Source: CAD feature listing. Evaluate the final solid. Frame: model axes, mm. Face numbers are marked on the shaded views. A direction names the side the tool comes from. Give positions to 0.01 mm unless a question says otherwise; leave off trailing zeros. Loops run counter-clockwise (first coordinate to the right, second up) from the corner with the lowest first, then second, coordinate; pieces in that order, holes last. Notation, with made-up numbers: (23.25, 0.25) -> (52.25, 0.25) arc R22 cw to (52.25, 8.25) -> close; hole circle Ø5 at (2.25, 69.5). An arc over 180 degrees is marked (long way). Return JSON: item names as keys, results as strings. Group by question number.
(1) Cut plane A-A on y = -11.9. Return loops of the section in (x, z) (3 decimals).
(2) Access query for the marked faces 1, 2 and 3. Directions: +Z, -Z, +X, -X, +Y, -Y. A direction counts if a zero-diameter tool reaches every point of the face in a straight line with its end or side. Return the directions, or none.
(3) Cut plane C-C on x = 2. Return loops of the section in (y, z).
(4) Cut plane B-B on z = 7. Return loops of the section in (x, y), then the cut area to 3 significant figures.
(5) Pin query (flat end, axial travel): pin 1 (3 mm diameter, centred on x = 3.5, z = 9, fed in from +Y); pin 2 (2.5 mm diameter, centred on x = 4.5, y = -11, fed in from -Z); pin 3 (4.5 mm diameter, centred on x = 3.925, y = -3.9, fed in from +Z); pin 4 (3 mm diameter, centred on y = -6.5, z = 9, fed in from +X). Return the tip coordinate at first contact, or that it passes through.
(6) Ray query, line 1 (X direction, y = -7.9, z = 0.75) (3 decimals); line 2 (X direction, y = -3.9, z = 2) (3 decimals); line 3 (Y direction, x = 6.25, z = 5.25). Return the intervals inside material, ascending. Write a range as from..to.
(7) Cut plane D-D on y = -7.9. Return loops of the section in (x, z) (3 decimals).
(8) Draft query along X for the marked faces 4, 5, 6 and 7. Return one class per face: released by +X, released by -X, zero draft, split by the parting line, or undercut.
Solid Edge part; units mm, degrees
sketch "Sketch1" plane through (0, 0, 0) normal (0, -1, 0) x (1, 0, 0)
  line L0 (0, 0) -> (0, 11.05)
  line L1 (7.85, 3.55) -> (2.9054, 11.802)
  line L2 (7.85, 0) -> (7.85, 3.55)
  line L3 (0, 0) -> (7.85, 0)
  arc A0 (0, 11.05) -> (2.9054, 11.802) centre (1.55, 11.05) cw
extrude "Protrusion1" add sketch "Sketch1" along normal blind 15.8
sketch "Sketch2" plane through (3.925, -14.4, 6.3) normal (0, -1, 0) x (1, 0, 0)
  line L0 (-3.925, -2.75) -> (-3.925, 4.75)
  line L1 (3.925, -2.75) -> (-3.925, -2.75)
  line L2 (-1.0196, 5.502) -> (3.925, -2.75)
  arc A0 (-1.0196, 5.502) -> (-3.925, 4.75) centre (-2.375, 4.75) cw
extrude "ExtrudedCutout_1" cut sketch "Sketch2" against normal blind 13
sketch "Sketch3" plane through (3.925, -7.9, 0) normal (0, 0, -1) x (0, 1, 0)
  line L0 (6.5, -2.405) -> (-6.5, -2.405)
  line L1 (-6.5, -2.405) -> (-6.5, 2.405)
  line L2 (-6.5, 2.405) -> (6.5, 2.405)
  line L3 (6.5, 2.405) -> (6.5, -2.405)
  circle A0 centre (0, 0) radius 1.4
  circle A1 centre (0, 0) radius 0.7
extrude "ExtrudedCutout_2" cut sketch "Sketch3" against normal blind 1.8
sketch "Sketch4" plane through (3.925, -7.9, 0) normal (0, 0, -1) x (0, 1, 0)
  circle A0 centre (-4, 0) radius 2.4
  circle A1 centre (4, 0) radius 2.4
extrude "ExtrudedCutout_3" cut sketch "Sketch4" against normal blind 2.1224
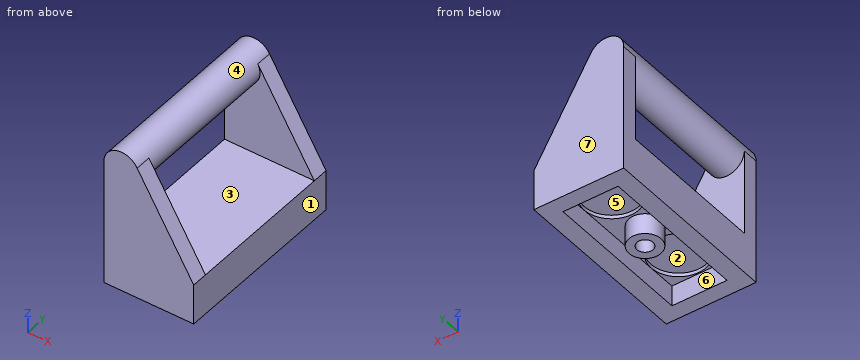
Answers:
{
 "1": {"outline": "(0, 0) -> (1.52, 0) -> (1.52, 1.8) -> (1.525, 1.8) -> (1.525, 2.122) -> (6.325, 2.122) -> (6.325, 1.8) -> (6.33, 1.8) -> (6.33, 0) -> (7.85, 0) -> (7.85, 3.55) -> (0, 3.55) -> close; circle Ø3.1 at (1.55, 11.05)"},
 "2": {"face 1": "+Z, -Z, +X, +Y, -Y", "face 2": "-Z", "face 3": "+X, -X"},
 "3": {"outline": "(-15.8, 0) -> (-14.4, 0) -> (-14.4, 1.8) -> (-13.33, 1.8) -> (-13.33, 2.12) -> (-10.47, 2.12) -> (-10.47, 1.8) -> (-5.33, 1.8) -> (-5.33, 2.12) -> (-2.47, 2.12) -> (-2.47, 1.8) -> (-1.4, 1.8) -> (-1.4, 0) -> (0, 0) -> (0, 12.53) -> (-15.8, 12.53) -> close; hole (-14.4, 3.55) -> (-1.4, 3.55) -> (-1.4, 9.57) -> (-14.4, 9.57) -> close"},
 "4": {"outline": "(0, -15.8) -> (5.78, -15.8) -> (5.78, -14.4) -> (0, -14.4) -> close; (0, -1.4) -> (5.78, -1.4) -> (5.78, 0) -> (0, 0) -> close", "area": "16.2 mm²"},
 "5": {"pin 1": "y = 0", "pin 2": "z = 2.12", "pin 3": "z = 12.59", "pin 4": "x = 3"},
 "6": {"line 1": "0..1.52, 2.525..3.225, 4.625..5.325, 6.33..7.85", "line 2": "0..1.525, 6.325..7.85", "line 3": "-15.8..-14.4, -1.4..0"},
 "7": {"outline": "(0, 0) -> (1.52, 0) -> (1.52, 1.8) -> (2.525, 1.8) -> (2.525, 0) -> (3.225, 0) -> (3.225, 1.8) -> (4.625, 1.8) -> (4.625, 0) -> (5.325, 0) -> (5.325, 1.8) -> (6.33, 1.8) -> (6.33, 0) -> (7.85, 0) -> (7.85, 3.55) -> (0, 3.55) -> close; circle Ø3.1 at (1.55, 11.05)"},
 "8": {"face 4": "split by the parting line", "face 5": "undercut", "face 6": "undercut", "face 7": "zero draft"}
}
